The figure shows three views and two pictorial views of one solid part (mm, origin at its lowest corner). Answer the questions. A direction names the side the tool comes from. Coordinates: 2 decimals unless noted, no trailing zeros. Write each loop counter-clockwise with the first axis right and the second up, starting at its lowest first coordinate (ties: lowest second). Pieces come first, ordered by that corner, then holes.
Item 1: Section B-B (x = 12) is taken. Give the vertices of the cut face in (y, z), then the cut area to 3 significant figures.
Item 2: Section A-A (y = 12) is taken. Give the vertices of the cut face in (x, z).
Item 3: Straight lines are drawn through the part: probe 1 along Z at (x, y) = (8.5, 33); probe 2 along X at (y, z) = (19, 19); probe 3 along Y at (x, z) = (16.5, 222). For each, find the intervals that lie inside material, in ascending order.
Item 4: Each of these flat-tipped pins is pushed along its axis until it touches: P1, Ø15, axis at x = 13, y = 11, coming from the -Z side; P2, Ø9.5, axis at x = 5, y = 25.5, coming from the +Z side; P3, Ø1, axis at x = 5, y = 32.5, coming from the -Z side. Where does it stop, or does it pass through?
Item 5: A tool of negligible diameter and unlimited length cuts with its end or side. For the marked faces 1, 2 and 3, from which of +Z, -Z, +X, -X, +Y, -Y can it reach the whole face along a straight path? Write none if from no direction.
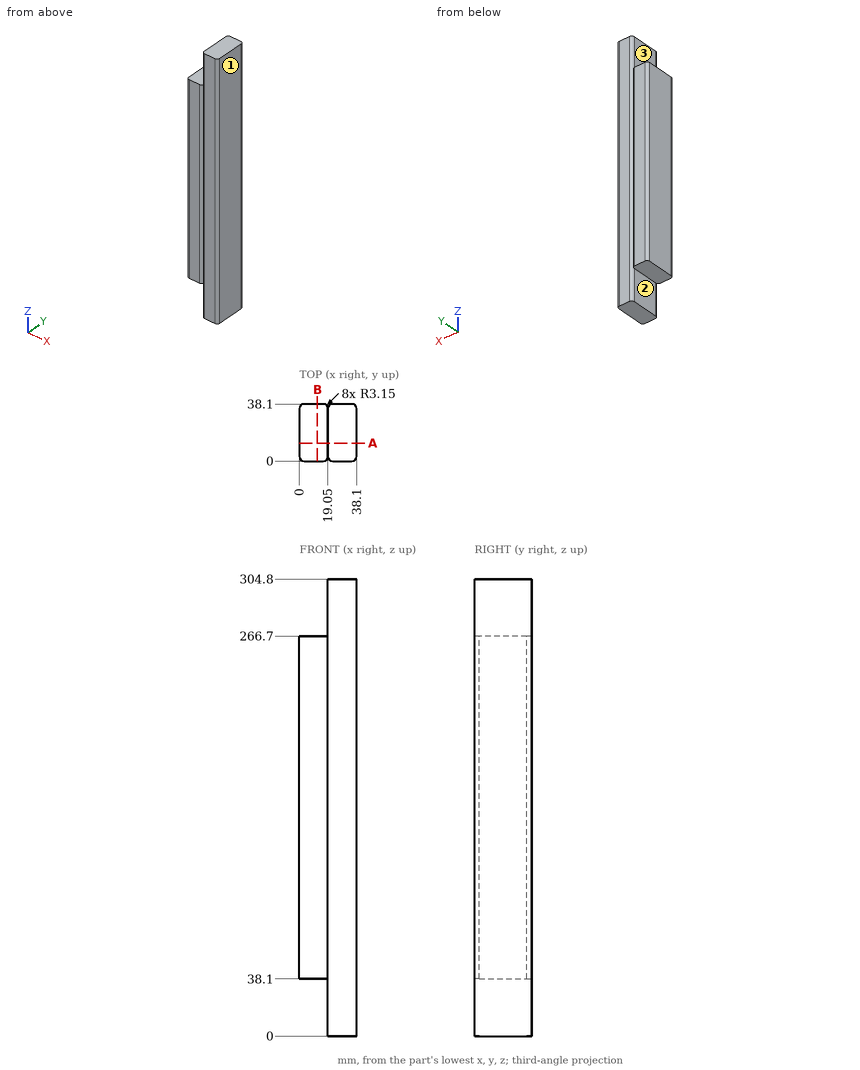
Established:
1. outline: (0, 38.1) - (38.1, 38.1) - (38.1, 266.7) - (0, 266.7) - close
1. area: 8,710 mm2
2. outline: (0, 38.1) - (19.05, 38.1) - (19.05, 0) - (38.1, 0) - (38.1, 304.8) - (19.05, 304.8) - (19.05, 266.7) - (0, 266.7) - close
3. probe 1: z = 38.1 to 266.7
3. probe 2: x = 19.05 to 38.1
3. probe 3: y = 0.06 to 38.04
4. P1: stops at z = 0
4. P2: stops at z = 266.7
4. P3: stops at z = 38.1
5. face 1: +Z, -Z, +X, +Y, -Y
5. face 2: -Z, -X, +Y, -Y
5. face 3: +Z, -X, +Y, -Y
